The listing builds one solid part. Answer for the finished solid, in the listing's coordinates (mm). A direction names the side the tool comes from. Give positions to 0.01 mm unless a question says otherwise; leave off trailing zeros. Loops run counter-clockwise (first coordinate to the right, second up) from the corner with the lowest first, then second, coordinate; pieces in that order, holes last. Notation, with made-up numbers: M 87,-10.75 L 123,-10.75 A17 cw 123,22.25 Z; hole C 56,-11 d4. An arc over 180 degrees is marked long. Return JSON: item names as keys, results as strings.
from build123d import *

# Parameters (mm, degrees)
F1_R     = 1.5875
F2_DEPTH = 25.4
F3_DEPTH = 12.7
F5_R     = 9.525
F5_R_2   = 1.5875
F6_DEPTH = 25.4


with BuildPart() as f2:
    # F1 (on Right) → F2 (new body, symmetric)
    with BuildSketch(Plane.YZ):
        with BuildLine():
            Line((-45.1303571429, -9.5006704583), (-0.9071428571, -12.6675606111))
            ThreePointArc((-0.9071428571, -12.6675606111), (12.7, 0), (-0.9071428571, 12.6675606111))
            Line((-0.9071428571, 12.6675606111), (-45.1303571429, 9.5006704583))
            ThreePointArc((-45.1303571429, 9.5006704583), (-53.975, 0), (-45.1303571429, -9.5006704583))
        make_face()
        with Locations((-44.45, 0)):
            Circle(F1_R, mode=Mode.SUBTRACT)
        Circle(F1_R, mode=Mode.SUBTRACT)
    extrude(amount=F2_DEPTH, both=True)

    # F0 (on Top) → F3 (intersect, symmetric)
    with BuildSketch(Plane.XY):
        with BuildLine():
            Line((6.0986519691, -46.6237074677), (13.1521007809, -9.5754071973))
            Line((13.1521007809, -9.5754071973), (5.969, 10.16))
            Line((5.969, 10.16), (3.4413070321, 9.3918339606))
            ThreePointArc((3.4413070321, 9.3918339606), (-2.998086321, 5.846793894), (-7.4532066327, 0))
            ThreePointArc((-7.4532066327, 0), (-8.6264344272, -3.2618802949), (-9.1444445756, -6.6894146861))
            Line((-9.1444445756, -6.6894146861), (-12.7, -44.45))
            ThreePointArc((-12.7, -44.45), (-4.2690955154, -53.9119543437), (6.0986519691, -46.6237074677))
        make_face()
    extrude(amount=F3_DEPTH, both=True, mode=Mode.INTERSECT)

    # F5 (on offset) → F6 (cut)
    with BuildSketch(Plane.YZ.offset(-3.175)):
        with Locations((-44.45, 0)):
            Circle(F5_R)
        with Locations((-44.45, 0)):
            Circle(F5_R_2, mode=Mode.SUBTRACT)
    extrude(amount=F6_DEPTH, mode=Mode.SUBTRACT)


solid = f2.part
(1) Straight lines are drawn through the part: line 1 along Y through (x, z) = (-6, 0); line 2 along Z through (x, y) = (-3.75, 0); line 3 along Y through (x, z) = (-6.25, 0). For each, find the intervals that lie inside material, in ascending order.
Values follow:
{"line 1": "-53.55 to -46.04, -42.86 to -1.59, 1.59 to 2.51", "line 2": "-12.7 to -1.59, 1.59 to 12.7", "line 3": "-53.46 to -46.04, -42.86 to -1.59, 1.59 to 2.14"}
(2) Given pin 1 (5 mm diameter, centred on y = -23, z = -8.5, fed in from +X); pin 2 (3 mm diameter, centred on y = -44.45, z = 0, fed in from +X); pin 3 (5 mm diameter, centred on x = 1.5, z = 5.5, fed in from +Y); pin 4 (6 mm diameter, centred on y = -8.5, z = 4, fed in from -X), each flat-ended and moving along its own axis, determine where each tip first touches the part or whether it passes through.
Values follow:
{"pin 1": "x = 11.07", "pin 2": "through", "pin 3": "y = 9.56", "pin 4": "x = -9.6"}
(3) The part is cut by section C-C (z = 4). Determine the outline of the cut face in (x, y) (3 decimals).
Values follow:
{"outline": "M -12.7,-44.45 A9.525 ccw -7.175,-53.094 L -3.175,-53.094 L -3.175,-35.806 L 8.158,-35.806 L 13.152,-9.575 L 5.969,10.16 L 3.441,9.392 A17.78 ccw -9.144,-6.689 Z"}
(4) The part is cut by section D-D (x = -4). Give the number of separate pieces and of enclosed holes in the cut face, and give its area (3 significant figures).
Values follow:
{"separate pieces": "1", "enclosed holes": "2", "area": "1,240 mm²"}
(5) A tool of negligible diameter and unlimited length cuts with its end or side. For faces 1 (the flat face through (-3.175, -45, -2)), 2 (the cylindrical face through (-11.036, -49.829, 0.134)), from which of +Z, -Z, +X, -X, +Y, -Y can it reach the whole face along a straight path? Write none if from no direction.
Values follow:
{"face 1": "+X, -Y", "face 2": "+Z, -Z, -X, -Y"}
(6) The part is cut by section A-A (y = 0). Determine the outline of the cut face in (x, z), and give its area (3 significant figures).
Values follow:
{"outline": "M -7.45,-12.7 L 9.67,-12.7 L 9.67,-1.59 L -7.45,-1.59 Z; M -7.45,1.59 L 9.67,1.59 L 9.67,12.7 L -7.45,12.7 Z", "area": "380 mm²"}
